Here's how the part is built. I have some questions about the finished solid (model axes, mm). Face numbers are marked on the shaded views. Give positions to 0.01 mm unless a question says otherwise; leave off trailing zeros. Loops run counter-clockwise (first coordinate to the right, second up) from the corner with the lowest first, then second, coordinate; pieces in that order, holes last.
Q1. Thinking about a two-plate mould opening in Y: for the marked faces 1, 2, 3 and 4, which applies, pulls with the +Y half, pulls with the -Y half, needs draft (parallel to the pull), parting line crosses it, or undercut?
Q2. Suppose I cut it at A-A (y = 0). List the corners of the cut face in (x, z) for me.
Q3. I need wall thicknesses on probe 1 along Y at (x, z) = (0, 3.1); probe 2 along Y at (x, z) = (2.5, 3.7); probe 3 along X at (y, z) = (-2.5, 0.75). Which ranges of each line are inside material? Lowest first, please.
Q4. Suppose I cut it at C-C (z = 2.2). List the corners of the cut face in (x, y) for me.
Q5. Suppose I cut it at B-B (x = 0). List the corners of the cut face in (y, z) for me, and give its area (3 significant figures).
Autodesk Fusion 360 part; units mm, degrees
sketch "Sketch1" plane through (0, 0, 0) normal (0, 0, 1) x (1, 0, 0)
  line L0 (6.5, -10) -> (-6.5, -10)
  line L1 (-6.5, -10) -> (-6.5, 10)
  line L2 (-6.5, 10) -> (6.5, 10)
  line L3 (6.5, 10) -> (6.5, -10)
  line L4 (6.5, -10) -> (-6.5, 10) construction
  line L5 (-6.5, -10) -> (6.5, 10) construction
  circle A0 centre (0, 0) radius 2.75
  dimension "d1" = 13
  dimension "d2" = 20
  dimension "d3" = 5.5
extrude "Extrude1" add sketch "Sketch1" along normal blind 6
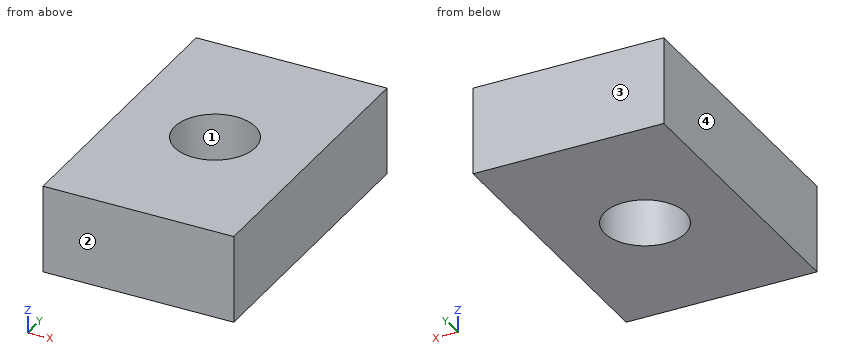
Solutions:
1. face 1: undercut
1. face 2: pulls with the -Y half
1. face 3: pulls with the +Y half
1. face 4: needs draft
2. outline: (-6.5, 0) - (-2.75, 0) - (-2.75, 6) - (-6.5, 6) - close; (2.75, 0) - (6.5, 0) - (6.5, 6) - (2.75, 6) - close
3. probe 1: y = -10 to -2.75, 2.75 to 10
3. probe 2: y = -10 to -1.15, 1.15 to 10
3. probe 3: x = -6.5 to -1.15, 1.15 to 6.5
4. outline: (-6.5, -10) - (6.5, -10) - (6.5, 10) - (-6.5, 10) - close; hole circle Ø5.5 at (0, 0)
5. outline: (-10, 0) - (-2.75, 0) - (-2.75, 6) - (-10, 6) - close; (2.75, 0) - (10, 0) - (10, 6) - (2.75, 6) - close
5. area: 87.0 mm2
